from build123d import *

# Parameters (mm, degrees)
SKETCH_1_W          = 88.07644651
SKETCH_1_H          = 60
EXTRUDE_1_DEPTH     = 3
SKETCH_2_R          = 2
CUT_EXTRUDE_1_DEPTH = 3
SKETCH_3_R          = 1.62
CUT_EXTRUDE_2_DEPTH = 3
SKETCH_4_R          = 3
CUT_EXTRUDE_3_DEPTH = 1


with BuildPart() as part:
    # 草图1 → 凸台-拉伸1 (new body)
    with BuildSketch(Plane.XY):
        with Locations((-120.442831111, 30)):
            Rectangle(SKETCH_1_W, SKETCH_1_H)
    extrude(amount=EXTRUDE_1_DEPTH)

    # 草图2 → 切除-拉伸1 (cut)
    with BuildSketch(Plane.XY.offset(3)):
        with Locations((-159.481054366, 5)):
            Circle(SKETCH_2_R)
        with Locations((-159.481054366, 55)):
            Circle(SKETCH_2_R)
        with Locations((-139.481054366, 5)):
            Circle(SKETCH_2_R)
        with Locations((-139.481054366, 55)):
            Circle(SKETCH_2_R)
        with Locations((-81.404607856, 5)):
            Circle(SKETCH_2_R)
        with Locations((-81.404607856, 55)):
            Circle(SKETCH_2_R)
        with Locations((-101.404607856, 55)):
            Circle(SKETCH_2_R)
        with Locations((-101.404607856, 5)):
            Circle(SKETCH_2_R)
    extrude(amount=-CUT_EXTRUDE_1_DEPTH, mode=Mode.SUBTRACT)

    # 草图3 → 切除-拉伸2 (cut)
    with BuildSketch(Plane(origin=(0, 0, 0), x_dir=(-1, 0, 0), z_dir=(0, 0, -1))):
        with Locations((96.404607856, 36)):
            Circle(SKETCH_3_R)
        with Locations((96.404607856, 24)):
            Circle(SKETCH_3_R)
        with Locations((146.404607856, 36)):
            Circle(SKETCH_3_R)
        with Locations((146.404607856, 24)):
            Circle(SKETCH_3_R)
    extrude(amount=-CUT_EXTRUDE_2_DEPTH, mode=Mode.SUBTRACT)

    # 草图4 → 切除-拉伸3 (cut)
    with BuildSketch(Plane(origin=(0, 0, 0), x_dir=(-1, 0, 0), z_dir=(0, 0, -1))):
        with Locations((96.404607856, 36)):
            Circle(SKETCH_4_R)
        with Locations((96.404607856, 24)):
            Circle(SKETCH_4_R)
        with Locations((146.404607856, 36)):
            Circle(SKETCH_4_R)
        with Locations((146.404607856, 24)):
            Circle(SKETCH_4_R)
    extrude(amount=-CUT_EXTRUDE_3_DEPTH, mode=Mode.SUBTRACT)


solid = part.part
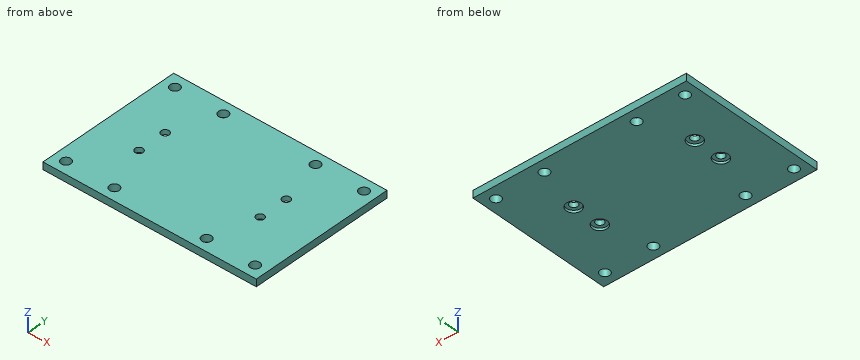
The model under review builds one solid part; all positions refer to its coordinate system, in mm. Round coordinates to 2 decimals unless told otherwise and drop trailing zeros. Write each loop counter-clockwise with the first axis right and the second up, starting at its lowest first coordinate (ties: lowest second). Pieces come first, ordered by that corner, then holes. Notation, with made-up numbers: (-17.5, 85) -> (8.5, 85) arc R34 ccw to (8.5, 121) -> close; hole circle Ø5 at (-9, -6.75). An arc over 180 degrees is marked (long way). Answer as a JSON object with one key per item and string values.
1. We need section B-B on z = 1.6. State how many separate pieces and enclosed holes the cut face has, and give its area (3 significant figures).
Results found:
{"separate pieces": "1", "enclosed holes": "12", "area": "5,150 mm^2"}
2. Clearance check with flat-ended pins moving along their axes: pin 1 (5 mm diameter, centred on x = -96.4, y = 36, fed in from -Z); pin 2 (3 mm diameter, centred on x = -146.4, y = 24, fed in from +Z). State where each tip first meets the part, or that it passes through.
Results found:
{"pin 1": "stops at z = 1", "pin 2": "passes through"}
3. We need section C-C on y = 55. State the section outline as (x, z) points.
Results found:
{"outline": "(-164.48, 0) -> (-161.48, 0) -> (-161.48, 3) -> (-164.48, 3) -> close; (-157.48, 0) -> (-141.48, 0) -> (-141.48, 3) -> (-157.48, 3) -> close; (-137.48, 0) -> (-103.4, 0) -> (-103.4, 3) -> (-137.48, 3) -> close; (-99.4, 0) -> (-83.4, 0) -> (-83.4, 3) -> (-99.4, 3) -> close; (-79.4, 0) -> (-76.4, 0) -> (-76.4, 3) -> (-79.4, 3) -> close"}
4. We need section A-A on y = 36. State the section outline as (x, z) points.
Results found:
{"outline": "(-164.48, 0) -> (-149.4, 0) -> (-149.4, 1) -> (-148.02, 1) -> (-148.02, 3) -> (-164.48, 3) -> close; (-144.78, 1) -> (-143.4, 1) -> (-143.4, 0) -> (-99.4, 0) -> (-99.4, 1) -> (-98.02, 1) -> (-98.02, 3) -> (-144.78, 3) -> close; (-94.78, 1) -> (-93.4, 1) -> (-93.4, 0) -> (-76.4, 0) -> (-76.4, 3) -> (-94.78, 3) -> close"}
5. To check wall thickness, follow line 1 along Y through (x, z) = (-101.5, 0.25); line 2 along X through (y, z) = (6, 1.75); line 3 along Y through (x, z) = (-140, 2.3). State the ranges of each line that lie inside material, in increasing order.
Results found:
{"line 1": "y = 0 to 3, 7 to 53, 57 to 60", "line 2": "x = -164.48 to -161.21, -157.75 to -141.21, -137.75 to -103.14, -99.67 to -83.14, -79.67 to -76.4", "line 3": "y = 0 to 3.07, 6.93 to 53.07, 56.93 to 60"}
